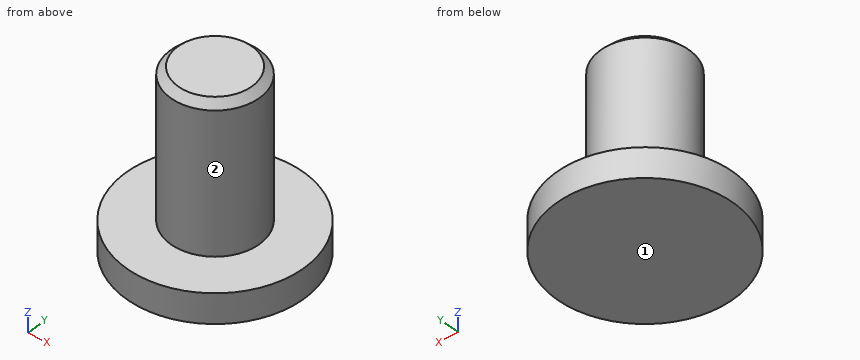
Autodesk Inventor part; units mm, degrees
ref_plane "YZ Plane" through (0, 0, 0) normal (1, 0, 0) x (0, 1, 0)
ref_plane "XZ Plane" through (0, 0, 0) normal (0, 1, 0) x (-1, 0, 0)
ref_plane "XY Plane" through (0, 0, 0) normal (0, 0, 1) x (1, 0, 0)
sketch "Sketch1" plane through (0, 0, 0) normal (0, 0, 1) x (1, 0, 0)
  circle A0 centre (0, 0) radius 6
  dimension "d0" = 12
extrude "Extrusion1" add sketch "Sketch1" along normal blind 2
sketch "Sketch2" plane through (0, 0, 2) normal (0, 0, 1) x (1, 0, 0)
  circle A0 centre (0, 0) radius 3
  dimension "d3" = 6
extrude "Extrusion2" add sketch "Sketch2" along normal blind 10
chamfer "Chamfer1" distance 0.5 angle 45 1 edges at (-3, 0, 12)
properties part number "pin"
Here's how the part is built. I have some questions about the finished solid (model axes, mm). Face numbers are marked on the shaded views. A direction names the side the tool comes from. Coordinates: 2 decimals unless noted, no trailing zeros. Loops run counter-clockwise (first coordinate to the right, second up) from the corner with the lowest first, then second, coordinate; pieces in that order, holes last.
1. For P1, Ø3, axis at y = -3.5, z = 7, coming from the -X side; P2, Ø3, axis at y = -1.5, z = 9, coming from the -X side; P3, Ø2, axis at x = 3.5, z = 8.5, coming from the +Y side, each with a flat end and sliding along its axis, tell me the tip position at first contact or that it passes through.
2. Imagine slicing it at A-A, the plane y = 0. Please give me the cut outline in (x, z), and give its area (4 significant figures).
3. For the marked faces 1 and 2, which set-ups out of +Z, -Z, +X, -X, +Y, -Y let a thin tool reach every point of the face, with its end or its side?
4. Imagine slicing it at D-D, the plane y = -4.5. Please give me the cut outline in (x, z), and give its area (3 significant figures).
5. Imagine slicing it at C-C, the plane z = 5.25. Please give me the cut outline in (x, y).
6. I need wall thicknesses on L1, parallel to Z at x = 2.25, y = -2.25; L2, parallel to X at y = 2.25, z = 9; L3, parallel to Y at x = 1, z = 10.5. Which ranges of each line are inside material? Lowest first, please.
Taken from the geometry:
1. P1: stops at x = -2.24
1. P2: stops at x = -3
1. P3: stops at y = 1.66
2. outline: (-6, 0) - (6, 0) - (6, 2) - (3, 2) - (3, 11.5) - (2.5, 12) - (-2.5, 12) - (-3, 11.5) - (-3, 2) - (-6, 2) - close
2. area: 83.75 mm2
3. face 1: -Z, +X, -X, +Y, -Y
3. face 2: +Z
4. outline: (-3.97, 0) - (3.97, 0) - (3.97, 2) - (-3.97, 2) - close
4. area: 15.9 mm2
5. outline: circle Ø6 at (0, 0)
6. L1: z = 0 to 2
6. L2: x = -1.98 to 1.98
6. L3: y = -2.83 to 2.83
